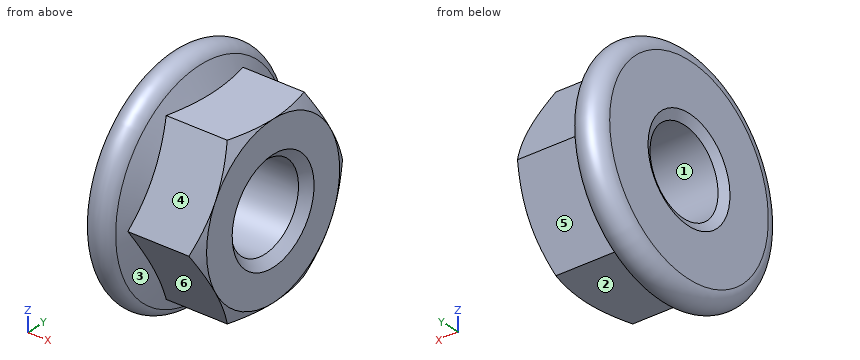
Autodesk Inventor part; units mm, degrees
ref_plane "Work Plane1" through (26.5484, 0, 0) normal (0, 0, -1) x (-1, 0, 0)
ref_plane "YZ Plane" through (0, 0, 0) normal (1, 0, 0) x (0, 1, 0)
ref_plane "XZ Plane" through (0, 0, 0) normal (0, 1, 0) x (-1, 0, 0)
sketch "Sketch1" plane through (0, 0, 0) normal (0, 0, 1) x (1, 0, 0)
  line L0 (-1.8442, 0) -> (9.6407, 0)
  line L1 (3.1069, 6.5) -> (2.2876, 8.2571)
  line L2 (3.1069, 6.5) -> (8, 6.5) construction
  line L3 (8, 6.5) -> (8, 0) construction
  arc A0 (2.2876, 8.2571) -> (0, 7.75) centre (1.2, 7.75) ccw
  line L4 (3.1069, 6.5) -> (3.1069, 0)
  line L5 (0, -1.835) -> (0, 11.0102)
  point P0 (0, 0)
  dimension "d2" = 13
  dimension "d4" = 17.9
  dimension "d5" = 1.2
  dimension "d15" = 8
  dimension "d16" = 25
revolve "Ring" add sketch "Sketch1" angle 360 about axis through (-10, 0, 0) along (1, 0, 0)
sketch "Sketch2" plane through (0, 0, 0) normal (-1, 0, 0) x (0, 0, 1)
  circle A0 centre (0, 0) radius 4.9
  line L0 (-6.5, -3.7528) -> (-6.5, 3.7528)
  line L1 (-6.5, 3.7528) -> (0, 7.5056)
  line L2 (0, 7.5056) -> (6.5, 3.7528)
  line L3 (6.5, 3.7528) -> (6.5, -3.7528)
  line L4 (6.5, -3.7528) -> (0, -7.5056)
  line L5 (0, -7.5056) -> (-6.5, -3.7528)
  circle A1 centre (0, 0) radius 7.75
  dimension "d6" = 15.0111
extrude "Body" add sketch "Sketch2" against normal blind 8 contours A0 | L0 L1 L2 L3 L4 L5
sketch "Sketch3" plane through (0, 0, 0) normal (0, 0, 1) x (1, 0, 0)
  line L0 (2.638, 7.5056) -> (8, 7.5056)
  line L1 (8, 3.7528) -> (8, 7.5056)
  line L2 (0, -7.75) -> (0, 7.75)
  line L3 (-1.6, 0) -> (9.6, 0)
  line L4 (7.4194, 7.5056) -> (8, 6.5)
  dimension "d10" = 30
  dimension "d11" = 13
revolve "Chamfer1" cut sketch "Sketch3" angle 360 about axis through (-10, 0, 0) along (1, 0, 0)
sketch "Sketch4" plane through (0, 0, 0) normal (-1, 0, 0) x (0, 0, 1)
  circle A0 centre (0, 0) radius 7.75
hole "Thread" at (0, 0, 0) direction (1, 0, 0) diameter 6.647 end through all
chamfer "Chamfer2" distance 0.6766 angle 30 1 edges at (0, 0, -3.3235) measured on face at (0, 6.1914, -0.7518)
ref_plane "Work Plane1" through (26.5484, 0, 0) normal (0, 0, -1) x (-1, 0, 0)
chamfer "Chamfer3" distance 0.6766 angle 45 1 edges at (8, 0, -3.3235)
equation "\"d2\" = SW"
equation "\"d4\" = LADI"
equation "\"d5\" = PHH"
equation "\"d15\" = KOH"
equation "\"d16\" = KEWI"
equation "\"d6\" = 1.1547 * SW"
equation "\"d7\" = KOH"
equation "\"d10\" = ANG1"
equation "\"d11\" = SW0"
equation "\"d12\" = -0.5 * GD1 + 0.5 * NND"
equation "\"d46\" = -0.5 * GD1 + 0.5 * NND"
equation "\"d51\" = -0.5 * GD1 + 0.5 * NND"
equation "\"ANG1\" = 30deg"
equation "\"KEWI\" = 25deg"
equation "\"NND\" = 8"
equation "\"LADI\" = 17.9"
equation "\"SW\" = 13"
equation "\"PHH\" = 1.2"
equation "\"KOH\" = NND"
equation "\"SW0\" = 13"
equation "\"d1\" = LADI"
equation "\"d3\" = PHH"
equation "\"GUL\" = 0.541266 * PTC"
equation "\"RR\" = PHH"
equation "\"THREADDIA\" = 8"
equation "\"TOA\" = 30deg"
equation "\"PTC\" = 1.25"
equation "\"GAL\" = 0.541266 * PTC"
equation "\"E0\" = 1.155 * SW"
properties part number "ISO 4161 - M8(1)" material "Stainless Steel"
Could you check a few things on this model? Use its own coordinates, in mm. Face numbers are marked on the shaded views. A direction names the side the tool comes from. Give positions to 0.01 mm unless a question says otherwise; leave off trailing zeros. Order: outer loops, then holes, each group sorted by start corner. A loop starts at its lowest first (then second) coordinate and runs counter-clockwise, first axis right, second up. Notation, with made-up numbers: (-9, 20.25) - (17, 20.25) arc R30 ccw to (17, 52.25) - close; hole circle Ø9 at (82.5, -25.75). An arc over 180 degrees is marked (long way). One line per item, written item: value. Start each with the question number.
1. If I drill on probe 1 along Z at (x, y) = (4.75, 0); probe 2 along X at (y, z) = (-6.5, -3.75); probe 3 along Z at (x, y) = (5.25, -1.25), over which ranges is the centre line in solid material (lowest first)?
2. For the marked faces 4, 5 and 6, which set-ups out of +Z, -Z, +X, -X, +Y, -Y let a thin tool reach every point of the face, with its end or its side?
3. Imagine slicing it at A-A on x = 6.75. List the corners of the cut face in (y, z) for me, plus the area to 3 significant figures.
4. Thinking about a two-plate mould opening in Y: for the marked faces 1, 2 and 3, which applies, +Y half, -Y half, draft (parallel to the pull), parting line (faces both ways), or undercut?
5. Imagine slicing it at B-B on x = 1.5. List the corners of the cut face in (y, z) for me, plus the area to 3 significant figures.
6. For P1, Ø2, axis at y = -7, z = 0.5, coming from the +X side; P2, Ø2, axis at x = 5, z = 0.5, coming from the -Y side; P3, Ø2.5, axis at x = 4.5, y = -2, coming from the -Z side; P4, Ø3, axis at x = 6.5, z = -7, coming from the -Y side, each with a flat end and sliding along its axis, tell me the tip position at first contact or that it passes through.
Values:
1. probe 1: -6.5 to -3.32, 3.32 to 6.5
1. probe 2: 0 to 2.64
1. probe 3: -6.5 to -3.08, 3.08 to 6.5
2. face 4: +Z, +X, -Y
2. face 5: -Z, +X, +Y
2. face 6: -Z, +X, -Y
3. outline: (-7.51, 0) - (-3.75, -6.5) - (3.75, -6.5) - (7.51, 0) - (3.75, 6.5) - (-3.75, 6.5) - close; hole circle Ø6.65 at (0, 0)
3. area: 112 mm²
4. face 1: undercut
4. face 2: draft
4. face 3: parting line
5. outline: circle Ø17.82 at (0, 0); hole circle Ø6.65 at (0, 0)
5. area: 215 mm²
6. P1: x = 8
6. P2: y = -7.51
6. P3: z = -6.5
6. P4: y = -4.33
